Source: CAD feature listing. Evaluate the final solid. Frame: model axes, mm. A direction names the side the tool comes from. Round coordinates to 2 decimals unless told otherwise and drop trailing zeros. Loops run counter-clockwise (first coordinate to the right, second up) from the corner with the lowest first, then second, coordinate; pieces in that order, holes last. Notation, with made-up numbers: M 43,33 L 73,33 A29 ccw 73,64 Z; hole C -24.5,-11 d7. An arc over 180 degrees is marked long. Write each question's results on one line, items separated by ' | '. Start each with the question number.
1. Draft query along X for faces 1 (the flat face through (9, 25, 1)), 2 (the flat face through (-19, 1, 1)), 3 (the cylindrical face through (-23, 10, 1)). Return one class per face: released by +X, released by -X, zero draft, split by the parting line, or undercut.
2. Set-up query: faces 4 (the flat face through (-9, -5, 1)), 5 (the flat face through (19, 19, 1)), 6 (the flat face through (9, -4, 1)). Return all of +Z, -Z, +X, -X, +Y, -Y with unobstructed straight access to the full face (end or side cutting, diameter ignored); none if empty.
3. Section D-D on y = 10. Output: boundary loops of the cut face in (x, z).
4. Contact query for flat-ended pins moving along their axis: pin 1 Ø1 at (x, z) = (23.5, 1) entering from +Y; pin 2 Ø0.6 at (y, z) = (24, 1.5) entering from +X; pin 3 Ø1 at (x, z) = (-16, 0.5) entering from -Y. Output: stop coordinate, or through.
5. Section C-C on z = 0.4. Give the number of separate pieces and of enclosed holes in the cut face, and give its area (3 significant figures).
6. Ray query, line 1 (Y direction, x = 10, z = 0.7); line 2 (Y direction, x = 0, z = 0.6); line 3 (Y direction, x = -1, z = 1.6). Return the intervals inside material, ascending.
7. Section A-A on x = 0. Output: boundary loops of the cut face in (y, z).
8. Section B-B on x = -20. Output: boundary loops of the cut face in (y, z).
from build123d import *

# Parameters (mm, degrees)
SKETCH_1_R      = 3
EXTRUDE_1_DEPTH = 2


with BuildPart() as part:
    # 草图1 → 凸台-拉伸1 (new body)
    with BuildSketch(Plane.XY):
        with BuildLine():
            Line((-9, -9), (-9, 0))
            ThreePointArc((-9, 0), (-9.292893219, 0.707106781), (-10, 1))
            Line((-10, 1), (-29, 1))
            ThreePointArc((-29, 1), (-29.707106781, 1.292893219), (-30, 2))
            Line((-30, 2), (-30, 18))
            ThreePointArc((-30, 18), (-29.707106781, 18.707106781), (-29, 19))
            Line((-29, 19), (-10, 19))
            ThreePointArc((-10, 19), (-9.292893219, 19.292893219), (-9, 20))
            Line((-9, 20), (-9, 29))
            ThreePointArc((-9, 29), (-8.707106781, 29.707106781), (-8, 30))
            Line((-8, 30), (8, 30))
            ThreePointArc((8, 30), (8.707106781, 29.707106781), (9, 29))
            Line((9, 29), (9, 20))
            ThreePointArc((9, 20), (9.292893219, 19.292893219), (10, 19))
            Line((10, 19), (29, 19))
            ThreePointArc((29, 19), (29.707106781, 18.707106781), (30, 18))
            Line((30, 18), (30, 2))
            ThreePointArc((30, 2), (29.707106781, 1.292893219), (29, 1))
            Line((29, 1), (10, 1))
            ThreePointArc((10, 1), (9.292893219, 0.707106781), (9, 0))
            Line((9, 0), (9, -9))
            ThreePointArc((9, -9), (8.707106781, -9.707106781), (8, -10))
            Line((8, -10), (-8, -10))
            ThreePointArc((-8, -10), (-8.707106781, -9.707106781), (-9, -9))
        make_face()
        with Locations((0, 20)):
            Circle(SKETCH_1_R, mode=Mode.SUBTRACT)
        Circle(SKETCH_1_R, mode=Mode.SUBTRACT)
        with Locations((-20, 10)):
            Circle(SKETCH_1_R, mode=Mode.SUBTRACT)
        with Locations((-10, 10)):
            Circle(SKETCH_1_R, mode=Mode.SUBTRACT)
        with Locations((20, 10)):
            Circle(SKETCH_1_R, mode=Mode.SUBTRACT)
        with Locations((10, 10)):
            Circle(SKETCH_1_R, mode=Mode.SUBTRACT)
    extrude(amount=EXTRUDE_1_DEPTH)


solid = part.part
Taken from the geometry:
1) face 1: released by +X | face 2: zero draft | face 3: undercut
2) face 4: +Z, -Z, -X, -Y | face 5: +Z, -Z, +X, +Y | face 6: +Z, -Z, +X, -Y
3) outline: M -30,0 L -23,0 L -23,2 L -30,2 Z; M -17,0 L -13,0 L -13,2 L -17,2 Z; M -7,0 L 7,0 L 7,2 L -7,2 Z; M 13,0 L 17,0 L 17,2 L 13,2 Z; M 23,0 L 30,0 L 30,2 L 23,2 Z
4) pin 1: y = 19 | pin 2: x = 9 | pin 3: y = 1
5) separate pieces: 1 | enclosed holes: 6 | area: 1,310 mm^2
6) line 1: 1 to 7, 13 to 19 | line 2: -10 to -3, 3 to 17, 23 to 30 | line 3: -10 to -2.83, 2.83 to 17.17, 22.83 to 30
7) outline: M -10,0 L -3,0 L -3,2 L -10,2 Z; M 3,0 L 17,0 L 17,2 L 3,2 Z; M 23,0 L 30,0 L 30,2 L 23,2 Z
8) outline: M 1,0 L 7,0 L 7,2 L 1,2 Z; M 13,0 L 19,0 L 19,2 L 13,2 Z
